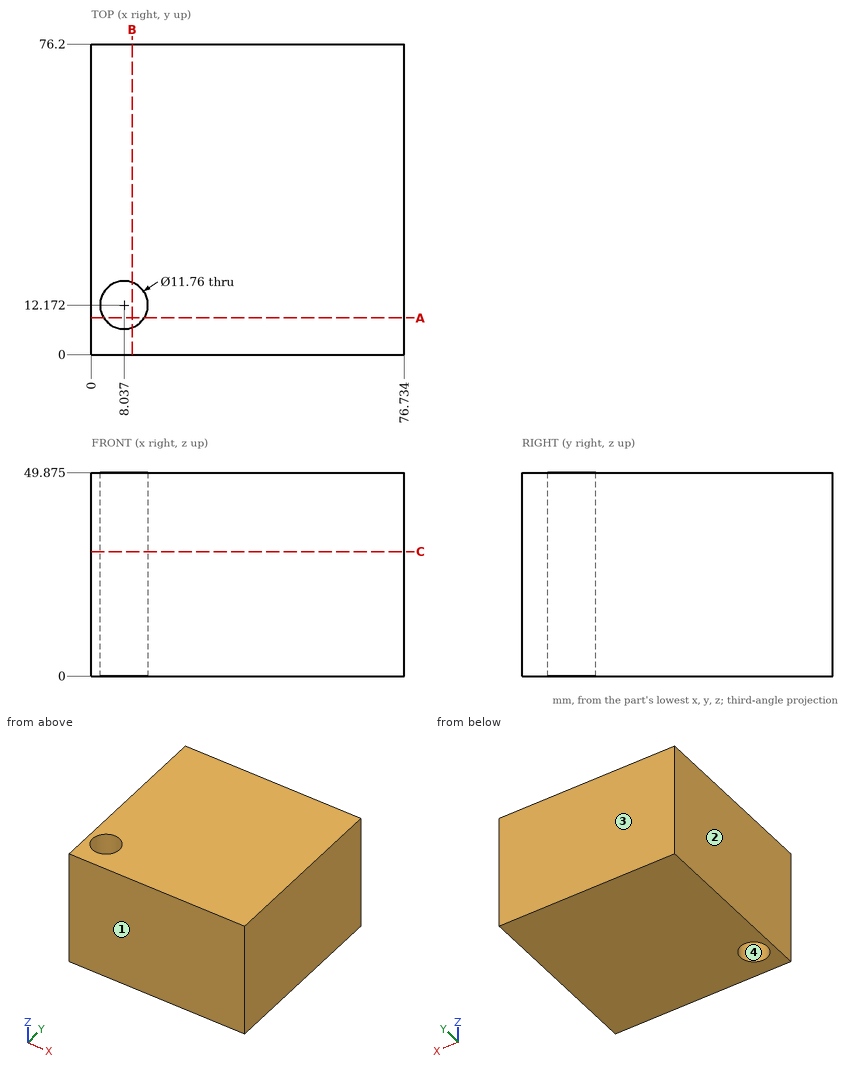
Drawing for the job (mm, zero at the part's lowest x, y, z). Give positions to 0.01 mm unless a question says otherwise; leave off trailing zeros. Order: outer loops, then holes, each group sorted by start corner. A loop starts at its lowest first (then second) coordinate and runs counter-clockwise, first axis right, second up. Notation, with made-up numbers: M 55,55 L 61,55 A15 cw 61,80 Z; hole C -8.5,57.25 d4. An arc over 180 degrees is marked long. Put each result on its own line as item: value.
Item 1: Probe line 1 (X direction, y = 10, z = 12.5) (1 decimal). List the from-to ranges inside material, lowest first. Write a range as [from, to].
From the geometry:
line 1: x = [0, 2.6], [13.5, 76.7]
Item 2: Slice it at C-C, the plane z = 30.5. Write the cut outline in (x, y) (1 decimal), plus the area to 3 significant figures.
From the geometry:
outline: M 0,0 L 76.7,0 L 76.7,76.2 L 0,76.2 Z; hole C 8,12.2 d11.8
area: 5,740 mm2
Item 3: Slice it at B-B, the plane x = 10. Write the cut outline in (y, z) (1 decimal), plus the area to 3 significant figures.
From the geometry:
outline: M 0,0 L 6.6,0 L 6.6,49.9 L 0,49.9 Z; M 17.7,0 L 76.2,0 L 76.2,49.9 L 17.7,49.9 Z
area: 3,250 mm2
Item 4: Two-plate mould, pull along Y, no slides. Class the marked faces 1, 2, 3 and 4: +Y half, -Y half, draft (parallel to the pull), parting line (faces both ways), or undercut.
From the geometry:
face 1: -Y half
face 2: draft
face 3: +Y half
face 4: undercut
Item 5: Flat gauge pins, fed straight in: pin 1 Ø12 at (y, z) = (10.5, 14.5) entering from -X; pin 2 Ø9.5 at (x, y) = (8.04, 12.17) entering from +Z. Where does each tip first touch, or does it go through?
From the geometry:
pin 1: stops at x = 0
pin 2: passes through
Item 6: Slice it at A-A, the plane y = 9. Write the cut outline in (x, z) (1 decimal).
From the geometry:
outline: M 0,0 L 3.1,0 L 3.1,49.9 L 0,49.9 Z; M 13,0 L 76.7,0 L 76.7,49.9 L 13,49.9 Z
